from build123d import *

# Parameters (mm, degrees)
SKETCH3_W           = 38.1
SKETCH3_H           = 38.1
BOSS_EXTRUDE2_DEPTH = 5.08
BOSS_EXTRUDE3_DEPTH = 1.27


with BuildPart() as part:
    # Sketch3 → Boss-Extrude2 (new body)
    with BuildSketch(Plane(origin=(0, 0, 0), x_dir=(1, 0, 0), z_dir=(0, 1, 0))):
        Rectangle(SKETCH3_W, SKETCH3_H)
    extrude(amount=-BOSS_EXTRUDE2_DEPTH)

    # Sketch2 → Boss-Extrude3 (add)
    with BuildSketch(Plane(origin=(0, 0, 0), x_dir=(1, 0, 0), z_dir=(0, 1, 0))):
        with BuildLine():
            Line((-17.562102448, 10.377897552), (-11.822643135, 4.638438239))
            ThreePointArc((-11.822643135, 4.638438239), (-12.7, 0), (-11.822643135, -4.638438239))
            Line((-11.822643135, -4.638438239), (-17.562102448, -10.377897552))
            ThreePointArc((-17.562102448, -10.377897552), (-17.562102448, -17.562102448), (-10.377897552, -17.562102448))
            Line((-10.377897552, -17.562102448), (-4.638438239, -11.822643135))
            ThreePointArc((-4.638438239, -11.822643135), (0, -12.7), (4.638438239, -11.822643135))
            Line((4.638438239, -11.822643135), (10.377897552, -17.562102448))
            ThreePointArc((10.377897552, -17.562102448), (17.562102448, -17.562102448), (17.562102448, -10.377897552))
            Line((17.562102448, -10.377897552), (11.822643135, -4.638438239))
            ThreePointArc((11.822643135, -4.638438239), (12.7, 0), (11.822643135, 4.638438239))
            Line((11.822643135, 4.638438239), (17.562102448, 10.377897552))
            ThreePointArc((17.562102448, 10.377897552), (17.562102448, 17.562102448), (10.377897552, 17.562102448))
            Line((10.377897552, 17.562102448), (4.638438239, 11.822643135))
            ThreePointArc((4.638438239, 11.822643135), (0, 12.7), (-4.638438239, 11.822643135))
            Line((-4.638438239, 11.822643135), (-10.377897552, 17.562102448))
            ThreePointArc((-10.377897552, 17.562102448), (-17.562102448, 17.562102448), (-17.562102448, 10.377897552))
        make_face()
    extrude(amount=BOSS_EXTRUDE3_DEPTH)


solid = part.part
The model under review builds one solid part; all positions refer to its coordinate system, in mm. A direction names the side the tool comes from. Round coordinates to 2 decimals unless told otherwise and drop trailing zeros. Order: outer loops, then holes, each group sorted by start corner. A loop starts at its lowest first (then second) coordinate and runs counter-clockwise, first axis right, second up. Notation, with made-up numbers: (9, 19.5) -> (44, 19.5) arc R20 ccw to (44, 56.5) -> close; hole circle Ø9 at (69.5, 77.25). An arc over 180 degrees is marked (long way). Use CSV: the item, a comma, the result in double quotes. Start each with the question number.
(1) Tool access review of faces 1 (the face through (0, 0, 16)), 2 (the face through (-14.652, 0.626, 7.468)), 3 (the face through (17.64, 0.63, -17.48)): name each direction out of +Z, -Z, +X, -X, +Y, -Y from which nothing blocks a thin tool from reaching the whole face with its end or side.
(2) Wall thickness on probe 1 along Z at (x, y) = (0.5, 0.75); probe 2 along Z at (x, y) = (17, 0.25); probe 3 along Y at (x, z) = (-13, 3): over which ranges is each line inside the solid? List them lowest first. Write a range as from..to.
(3) Consider section A-A on z = 6.5. Write out the cut boundary in (x, y), and give its area (3 significant figures).
(4) Consider section B-B on x = -8. Write out the cut boundary in (y, z), and give its area (3 significant figures).
(5) Insertion check: pin 1 (6 mm diameter, centred on x = 4.5, z = -17, fed in from +Y). The pin has a flat end and moves straight along its axis. Give the tip position at first contact, or say it passes through.
Responses:
1,face 1,"+Z, +Y"
1,face 2,"-X, +Y"
1,face 3,"+Y"
2,probe 1,"-12.69..12.69"
2,probe 2,"-18.05..-9.82, 9.82..18.05"
2,probe 3,"-5.08..0"
3,outline,"(-19.05, -5.08) -> (19.05, -5.08) -> (19.05, 0) -> (13.68, 0) -> (13.68, 1.27) -> (-13.68, 1.27) -> (-13.68, 0) -> (-19.05, 0) -> close"
3,area,"228 mm²"
4,outline,"(-5.08, -19.05) -> (0, -19.05) -> (0, -15.18) -> (1.27, -15.18) -> (1.27, 15.18) -> (0, 15.18) -> (0, 19.05) -> (-5.08, 19.05) -> close"
4,area,"232 mm²"
5,pin 1,"y = 0"
